Part model, mm, in its own coordinate system. A direction names the side the tool comes from. Round coordinates to 2 decimals unless told otherwise and drop trailing zeros. Write each loop counter-clockwise with the first axis right and the second up, starting at its lowest first coordinate (ties: lowest second). Pieces come first, ordered by that corner, then holes. Notation, with made-up numbers: M 70,7.5 L 74,7.5 A10 cw 74,14.5 Z; hole C 17.25,8 d7. An arc over 180 degrees is marked long. Use one line per item in the form item = value. Start each with the question number.
Item 1: Cut at C-C, the plane z = -13.5. Give the cut face in (x, y), then the cut area to 3 significant figures.
Item 2: Cut at D-D, the plane y = 0.5. Give the cut face in (x, z).
Item 3: Cut at A-A, the plane y = -7.5. Give the cut face in (x, z), then the cut area to 3 significant figures.
Item 4: Cut at B-B, the plane z = -29. Give the cut face in (x, y), then the cut area to 3 significant figures.
Item 5: Mould opens along X. For faces 6 (the face through (0, 1.2, 1)), 7 (the face through (-7.608, -3.616, 8.256)), 8 (the face through (11.67, 0.02, -12.81)), 9 (the face through (1, -7, 9)) say: +X half, -X half, draft (parallel to the pull), parting line (faces both ways), or undercut.
Item 6: Flat gauge pins, fed straight in: pin 1 Ø1.3 at (y, z) = (-2, -4.5) entering from -X; pin 2 Ø1.4 at (y, z) = (-8, 8) entering from +X; pin 3 Ø2 at (y, z) = (-3.5, 5) entering from -X; pin 4 Ø12 at (x, z) = (-8.5, -17.5) entering from -Y. Where does each tip first touch, or does it go through?
Item 7: Which spindle directions (+Z, -Z, +X, -X, +Y, -Y) get a long thin tool onto all of the face, cutting with end or side? Do faces 1 (the face through (3.5, -3.6, 6.2)), 2 (the face through (-17.43, 0.02, -24.11)), 3 (the face through (0, -3, 0)), 4 (the face through (-1, 0, 9)), 5 (the face through (3.15, -3.49, 9.24)). Say none if no direction does.
Item 8: Probe L1, parallel to X at y = 0.5, z = -3; L2, parallel to Y at x = 22, z = -27.5; L3, parallel to X at y = 0, z = -14. List the from-to ranges inside material, lowest first.
from build123d import *
from OCP.BRepFilletAPI import BRepFilletAPI_MakeChamfer

# Parameters (mm, degrees)
BOSS_EXTRUDE1_DEPTH      = 1.2
BOSS_EXTRUDE2_DEPTH      = 10
BOSS_EXTRUDE2_DEPTH_BACK = 2.2
SKETCH2_W                = 19.9
SKETCH2_H                = 9.5
CUT_EXTRUDE1_DEPTH       = 8
CUT_EXTRUDE2_DEPTH       = 42.835984366
CUT_EXTRUDE2_DEPTH_BACK  = 42.835984366
SKETCH4_W                = 8
SKETCH4_H                = 2
CHAMFER1_SIZE            = 2
CHAMFER2_SIZE            = 8
CHAMFER2_SIZE2           = 4.618802154


with BuildPart() as part:
    # Sketch1 → Boss-Extrude1 (new, symmetric)
    with BuildSketch(Plane(origin=(0, 0, 0), x_dir=(1, 0, 0), z_dir=(0, 1, 0))):
        Polygon((-7.75, 0), (0, 0), (0, -2.2), (-9.95, -2.2), (-9.95, 11.088730163), (-13.441735339, 14.580465501), (-25.639024707, 32), (-22.953320611, 32), (-11.75, 16), (-7.75, 12), align=None)
    boss_extrude1 = extrude(amount=BOSS_EXTRUDE1_DEPTH, both=True)

    # Mirror1: Boss-Extrude1 across plane
    add(boss_extrude1.mirror(Plane(origin=(0, 1.2, 0), x_dir=(0, 0, 1), z_dir=(-1, 0, 0))))

    # Sketch2 → Boss-Extrude2 (add, two sides: drawn at the far end of the back side and taken through both)
    with BuildSketch(Plane.XY.offset(2.2).offset(-BOSS_EXTRUDE2_DEPTH_BACK)):
        with Locations((0, -3.55)):
            Rectangle(SKETCH2_W, SKETCH2_H)
    extrude(amount=BOSS_EXTRUDE2_DEPTH + BOSS_EXTRUDE2_DEPTH_BACK)

    # Sketch3 → Cut-Extrude1 (cut)
    with BuildSketch(Plane.XY.offset(12.2)):
        with BuildLine():
            Line((-1, -0.562944594), (-1, 1.2))
            Line((-1, 1.2), (1, 1.2))
            Line((1, 1.2), (1, -0.562944594))
            ThreePointArc((1, -0.562944594), (3.15, -3.55), (1, -6.537055406))
            Line((1, -6.537055406), (1, -8.3))
            Line((1, -8.3), (-1, -8.3))
            Line((-1, -8.3), (-1, -6.537055406))
            ThreePointArc((-1, -6.537055406), (-3.15, -3.55), (-1, -0.562944594))
        make_face()
    extrude(amount=-CUT_EXTRUDE1_DEPTH, mode=Mode.SUBTRACT)

    # Sketch4 → Cut-Extrude2 (cut, two sides: drawn at the far end of the back side and taken through both)
    with BuildSketch(Plane(origin=(0, 0, 0), x_dir=(1, 0, 0), z_dir=(0, 1, 0)).offset(-CUT_EXTRUDE2_DEPTH_BACK)):
        with Locations((0, -5.2)):
            Rectangle(SKETCH4_W, SKETCH4_H)
    extrude(amount=CUT_EXTRUDE2_DEPTH + CUT_EXTRUDE2_DEPTH_BACK, mode=Mode.SUBTRACT)

    # Chamfer1
    chamfer1_edges = [part.edges().sort_by_distance(p)[0] for p in [
        (-8.85, -1.2, 0),
        (8.85, -1.2, 0),
    ]]
    chamfer(chamfer1_edges, length=CHAMFER1_SIZE)

    # Chamfer2: one chamfer whose edges measure the first distance from different faces: ONE call of the kernel's chamfer builder (chamfer() names one face for all edges)
    chamfer2_edges_1 = [part.edges().sort_by_distance(p)[0] for p in [
        (-9.95, -3.55, 12.2),
    ]]
    chamfer2_side_1 = [part.faces().sort_by_distance(p)[0] for p in [
        (-9.95, -2.87294894, 3.861970387),
    ]]
    chamfer2_edges_2 = [part.edges().sort_by_distance(p)[0] for p in [
        (9.95, -3.55, 12.2),
    ]]
    chamfer2_side_2 = [part.faces().sort_by_distance(p)[0] for p in [
        (9.95, -2.87294894, 3.861970387),
    ]]
    chamfer2 = BRepFilletAPI_MakeChamfer(part.part.solid().wrapped)
    for e in chamfer2_edges_1:
        chamfer2.Add(CHAMFER2_SIZE, CHAMFER2_SIZE2, e.wrapped, chamfer2_side_1[0].wrapped)  # the first distance lies on this face
    for e in chamfer2_edges_2:
        chamfer2.Add(CHAMFER2_SIZE, CHAMFER2_SIZE2, e.wrapped, chamfer2_side_2[0].wrapped)  # the first distance lies on this face
    add(Compound.cast(chamfer2.Shape()), mode=Mode.REPLACE)


solid = part.part
Model answer:
q1.outline = M -12.36,-1.2 L -9.25,-1.2 L -9.25,1.2 L -12.36,1.2 Z; M 9.25,-1.2 L 12.36,-1.2 L 12.36,1.2 L 9.25,1.2 Z
q1.area = 14.9 mm²
q2.outline = M -25.64,-32 L -22.95,-32 L -11.75,-16 L -7.75,-12 L -7.75,0 L 7.75,0 L 7.75,-12 L 11.75,-16 L 22.95,-32 L 25.64,-32 L 13.44,-14.58 L 9.95,-11.09 L 9.95,4.2 L 5.33,12.2 L 1,12.2 L 1,6.2 L 4,6.2 L 4,4.2 L -4,4.2 L -4,6.2 L -1,6.2 L -1,12.2 L -5.33,12.2 L -9.95,4.2 L -9.95,-11.09 L -13.44,-14.58 Z
q3.outline = M -9.95,0 L 9.95,0 L 9.95,4.2 L 5.33,12.2 L 1,12.2 L 1,6.2 L 4,6.2 L 4,4.2 L -4,4.2 L -4,6.2 L -1,6.2 L -1,12.2 L -5.33,12.2 L -9.95,4.2 Z
q3.area = 178 mm²
q4.outline = M -23.54,-1.2 L -20.85,-1.2 L -20.85,1.2 L -23.54,1.2 Z; M 20.85,-1.2 L 23.54,-1.2 L 23.54,1.2 L 20.85,1.2 Z
q4.area = 12.9 mm²
q5.face_6 = draft
q5.face_7 = -X half
q5.face_8 = +X half
q5.face_9 = undercut
q6.pin_1 = through
q6.pin_2 = 8.16
q6.pin_3 = -9.95
q6.pin_4 = -1.2
q7.face_1 = +Y, -Y
q7.face_2 = -Z, +Y, -Y
q7.face_3 = -Z, -Y
q7.face_4 = +Z, +Y, -Y
q7.face_5 = +Z
q8.L1 = -9.95 to -7.75, 7.75 to 9.95
q8.L2 = -1.2 to 1.2
q8.L3 = -12.86 to -9.75, 9.75 to 12.86
